Model file for the job. Use its own axes, mm. Face numbers are marked on the shaded views. A direction names the side the tool comes from. Round coordinates to 2 decimals unless told otherwise and drop trailing zeros. Loops run counter-clockwise (first coordinate to the right, second up) from the corner with the lowest first, then second, coordinate; pieces in that order, holes last. Notation, with made-up numbers: (12, 67.5) -> (23, 67.5) arc R19 ccw to (23, 98.5) -> close; hole circle Ø8 at (-24.75, -0.5). An arc over 180 degrees is marked (long way). Use a Markdown table: item, result.
from build123d import *

# Parameters (mm, degrees)
BOSS_EXTRUDE1_DEPTH = 13
SKETCH3_R           = 0.75
BOSS_EXTRUDE2_DEPTH = 1.4
FILLET1_R           = 0.2


with BuildPart() as part:
    # Sketch1 → Revolve1 (revolve)
    with BuildSketch(Plane.XY, mode=Mode.PRIVATE) as revolve1_sk:
        Polygon((0, 0), (0, 2), (-2, 1.272059531), (-2, 0), align=None)
    revolve(revolve1_sk.sketch.rotate(Axis((-2, 0, 0), (1, 0, 0)), 90), axis=Axis((-2, 0, 0), (1, 0, 0)))

    # Sketch2 → Boss-Extrude1 (add)
    with BuildSketch(Plane(origin=(0, 0, 0), x_dir=(0, 0, -1), z_dir=(1, 0, 0))):
        Polygon((0, 1.533333333), (-1.327905619, -0.766666667), (1.327905619, -0.766666667), align=None)
    extrude(amount=BOSS_EXTRUDE1_DEPTH)

    # Sketch3 → Boss-Extrude2 (add)
    with BuildSketch(Plane.ZY.offset(2)):
        Circle(SKETCH3_R)
    extrude(amount=BOSS_EXTRUDE2_DEPTH)

    # Fillet1
    fillet1_edges = [part.edges().sort_by_distance(p)[0] for p in [
        (6.5, -0.766666667, -1.327905619),
        (6.5, 1.533333333, 0),
        (6.5, -0.766666667, 1.327905619),
    ]]
    fillet(fillet1_edges, radius=FILLET1_R)


solid = part.part
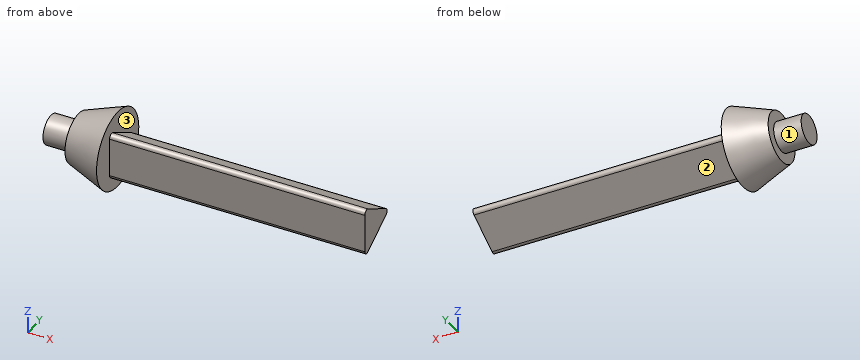
Q1. Band-saw the part on B-B, the plane x = 2.25. Give the cut face in (y, z), plus the area to 3 significant figures.
Results list:
| item | result |
|---|---|
| outline | (-0.77, -0.98) arc R0.2 ccw to (-0.47, -1.15) -> (1.23, -0.17) arc R0.2 ccw to (1.23, 0.17) -> (-0.47, 1.15) arc R0.2 ccw to (-0.77, 0.98) -> close |
| area | 2.97 mm² |
Q2. Band-saw the part on C-C, the plane y = 0. Give the cut face in (x, z), plus the area to 3 significant figures.
Results list:
| item | result |
|---|---|
| outline | (-3.4, -0.75) -> (-2, -0.75) -> (-2, -1.27) -> (0, -2) -> (0, -0.89) -> (13, -0.89) -> (13, 0.89) -> (0, 0.89) -> (0, 2) -> (-2, 1.27) -> (-2, 0.75) -> (-3.4, 0.75) -> close |
| area | 31.7 mm² |
Q3. Drill centre lines: L1, parallel to X at y = 1.1, z = 0; L2, parallel to X at y = 0.2, z = -1; L3, parallel to Y at x = 10.25, z = -0.45. Where is each one in solid material? Low to high. Write a range as from..to.
Results list:
| item | result |
|---|---|
| L1 | x = -2..13 |
| L2 | x = -2..0 |
| L3 | y = -0.77..0.75 |
Q4. Tool access for the marked faces 1, 2 and 3: list every direction of +Z, -Z, +X, -X, +Y, -Y with a clear straight run to the whole face (end or side of a thin tool).
Results list:
| item | result |
|---|---|
| face 1 | -X |
| face 2 | -Z, +X, +Y |
| face 3 | +X |
Q5. Flat gauge pins, fed straight in: pin 1 (2 mm diameter, centred on y = 1, z = 1.5, fed in from +X); pin 2 (1 mm diameter, centred on x = 3.5, z = -1, fed in from +Y); pin 3 (1 mm diameter, centred on x = 3.5, z = 0.5, fed in from -Y). Where does each tip first touch, or does it go through?
Results list:
| item | result |
|---|---|
| pin 1 | stops at x = 0 |
| pin 2 | stops at y = 0.67 |
| pin 3 | stops at y = -0.77 |
Q6. Band-saw the part on D-D, the plane x = -1.75. Give the cut face in (y, z), plus the area to 3 significant figures.
Results list:
| item | result |
|---|---|
| outline | circle Ø2.73 at (0, 0) |
| area | 5.84 mm² |
Q7. Band-saw the part on A-A, the plane z = 0. Give the cut face in (x, y), plus the area to 3 significant figures.
Results list:
| item | result |
|---|---|
| outline | (-3.4, -0.75) -> (-2, -0.75) -> (-2, -1.27) -> (0, -2) -> (0, -0.77) -> (13, -0.77) -> (13, 1.33) -> (0, 1.33) -> (0, 2) -> (-2, 1.27) -> (-2, 0.75) -> (-3.4, 0.75) -> close |
| area | 35.9 mm² |
